Geometry: final body of the model. Coordinates: model frame, mm. A direction names the side the tool comes from. Give positions to 0.01 mm unless a question says otherwise; leave off trailing zeros. Write each loop counter-clockwise with the first axis right and the second up, starting at its lowest first coordinate (ties: lowest second). Pieces come first, ordered by that corner, then holes. Notation, with made-up numbers: (77.25, 84.25) -> (102.25, 84.25) arc R23 cw to (102.25, 123.25) -> close; hole circle Ø9 at (84.25, -26.75). An arc over 180 degrees is marked (long way). Answer as a JSON object with one key per item and string values.
Autodesk Fusion 360 part; units mm, degrees
sketch "Skizze1" plane through (0, 0, 0) normal (0, 1, 0) x (1, 0, 0)
  line L0 (14.5, -1) -> (-13.5, -1)
  line L1 (-13.5, -1) -> (-13.5, 0)
  line L2 (-13.5, 0) -> (14.5, 0)
  line L3 (14.5, 0) -> (14.5, -1)
  line L4 (14.5, -1) -> (-13.5, 0) construction
  line L5 (-13.5, -1) -> (14.5, 0) construction
  line L6 (-13.5, 0) -> (-12.5, 0)
  line L7 (-12.5, 0) -> (-12.5, -7.5)
  line L8 (-12.5, -7.5) -> (-13.5, -7.5)
  line L9 (-13.5, -7.5) -> (-13.5, 0)
  line L10 (14.5, 0) -> (13.5, 0)
  line L11 (13.5, 0) -> (13.5, -7.5)
  line L12 (13.5, -7.5) -> (14.5, -7.5)
  line L13 (14.5, -7.5) -> (14.5, 0)
  line L14 (-12.5, -7.5) -> (-16.15, -7.5)
  line L15 (-16.15, -7.5) -> (-16.15, -6.5)
  line L16 (-16.15, -6.5) -> (-12.5, -6.5)
  line L17 (-12.5, -6.5) -> (-12.5, -7.5)
  line L18 (13.5, -7.5) -> (17.15, -7.5)
  line L19 (17.15, -7.5) -> (17.15, -6.5)
  line L20 (17.15, -6.5) -> (13.5, -6.5)
  line L21 (13.5, -6.5) -> (13.5, -7.5)
  point P0 (0.5, -0.5)
  dimension "d7" = 28
  dimension "d8" = 1
  dimension "d9" = 7.5
  dimension "d10" = 1
  dimension "d11" = 7.5
  dimension "d12" = 1
  dimension "d13" = 3.65
  dimension "d14" = 1
  dimension "d15" = 3.65
  dimension "d16" = 1
extrude "Extrusion1" add sketch "Skizze1" along normal blind 200
fillet "Abrundung1" radius 1.5 4 edges at (13.5, 100, 7.5) (-12.5, 100, 7.5) (14.5, 100, 0) (-13.5, 100, 0)
fillet "Abrundung2" radius 0.5 4 edges at (-13.5, 100, 6.5) (14.5, 100, 6.5) (13.5, 100, 1) (-12.5, 100, 1)
sketch "Skizze2" plane through (0, 0, 1) normal (0, 0, 1) x (-1, 0, 0)
  line L0 (12, -200) -> (12, 0)
  line L1 (12, 0) -> (-13, 0)
  line L2 (-13, 0) -> (-13, -200)
  line L3 (-13, -200) -> (12, -200)
  line L4 (0, 0) -> (0, -4.15) construction
  line L5 (-2.05, -6.2) -> (-2.05, -13.8)
  arc A0 (-2.05, -13.8) -> (2.05, -13.8) centre (0, -13.8) ccw
  line L6 (2.05, -13.8) -> (2.05, -6.2)
  arc A1 (2.05, -6.2) -> (-2.05, -6.2) centre (0, -6.2) ccw
  line L7 (0, -4.15) -> (0, -15.85) construction
  point P0 (0, -4.15)
  dimension "d26" = 4.15
  dimension "d34" = 11.7
  dimension "d35" = 4.1
extrude "Extrusion2" cut sketch "Skizze2" against normal blind 1 contours L5 A0 L6 A1
pattern_linear "R-Anordnung1" count 10 spacing 20 along (0, 1, 0) of "Extrusion2"
equation "InnerWidth = 28 mm"
equation "OuterWidth = 35.3 mm"
equation "Height = 7.5 mm"
equation "Thickness = 1 mm"
equation "Length = 200 mm"
equation "SlotDistance = 25 mm"
equation "d7 = InnerWidth"
equation "d8 = Thickness"
equation "d9 = Height"
equation "d10 = Thickness"
equation "d11 = Height"
equation "d12 = Thickness"
equation "d13 = ( OuterWidth - InnerWidth ) / 2"
equation "d14 = Thickness"
equation "d15 = ( OuterWidth - InnerWidth ) / 2"
equation "d16 = Thickness"
equation "d17 = Length"
equation "OuterFillet = 1.5 mm"
equation "d20 = OuterFillet"
equation "InnerFillet = OuterFillet - Thickness"
equation "d22 = InnerFillet"
equation "SlotWidth = 4.1 mm"
equation "SlotLength = 11.7 mm"
equation "SlotDistance2 = 20 mm"
equation "d26 = Linear Dimension-2"
equation "d30 = Length / SlotDistance2"
equation "d32 = SlotDistance2"
equation "d34 = SlotLength"
equation "d35 = SlotWidth"
Q1. Cut plane B-B (y = 42). Return the cut outline in (x, z).
Values:
{"outline": "(-16.15, 6.5) -> (-14, 6.5) arc R0.5 cw to (-13.5, 6) -> (-13.5, 1.5) arc R1.5 ccw to (-12, 0) -> (13, 0) arc R1.5 ccw to (14.5, 1.5) -> (14.5, 6) arc R0.5 cw to (15, 6.5) -> (17.15, 6.5) -> (17.15, 7.5) -> (15, 7.5) arc R1.5 ccw to (13.5, 6) -> (13.5, 1.5) arc R0.5 cw to (13, 1) -> (-12, 1) arc R0.5 cw to (-12.5, 1.5) -> (-12.5, 6) arc R1.5 ccw to (-14, 7.5) -> (-16.15, 7.5) -> close"}
Q2. Cut plane A-A (z = 4.75). Return the cut outline in (x, y), and give its area (3 significant figures).
Values:
{"outline": "(-13.5, 0) -> (-12.5, 0) -> (-12.5, 200) -> (-13.5, 200) -> close; (13.5, 0) -> (14.5, 0) -> (14.5, 200) -> (13.5, 200) -> close", "area": "400 mm²"}
Q3. Material intervals for L1, parallel to X at y = 106, z = 3; L2, parallel to Z at x = 12, y = 126.5; L3, parallel to Z at x = -14, y = 78, sorted ascending. Write a range as from..to.
Values:
{"L1": "-13.5..-12.5, 13.5..14.5", "L2": "0..1", "L3": "6.5..7.5"}
Q4. Cut plane C-C (x = -9). Return the cut outline in (y, z), and give its area (3 significant figures).
Values:
{"outline": "(0, 0) -> (200, 0) -> (200, 1) -> (0, 1) -> close", "area": "200 mm²"}
Q5. Set-up query: faces 1 (the flat face through (0.4, 0, 0.7)), 2 (the flat face through (14.5, 99, 4)), 3 (the flat face through (1, 99, 1)). Return all of +Z, -Z, +X, -X, +Y, -Y with unobstructed straight access to the full face (end or side cutting, diameter ignored); none if empty.
Values:
{"face 1": "+Z, -Z, +X, -X, -Y", "face 2": "-Z, +X, +Y, -Y", "face 3": "+Z, +Y, -Y"}
Q6. Cut plane D-D (x = 0). State how many separate pieces and enclosed holes the cut face has, and give its area (3 significant figures).
Values:
{"separate pieces": "11", "enclosed holes": "0", "area": "83.0 mm²"}
Q7. First-contact query: P1, Ø0.8, axis at y = 51.5, z = 0.5, coming from the -X side; P2, Ø1.7, axis at x = -15.5, y = 62.5, coming from the -Z side; P3, Ø0.5, axis at y = 91, z = 0.5, coming from the -X side; P4, Ø12, axis at x = 3.5, y = 58, coming from the -Z side. Flat tips, straight axial feed; report the tip coordinate or a pass-through.
Values:
{"P1": "x = -13.37", "P2": "z = 6.5", "P3": "x = -13.3", "P4": "z = 0"}
Q8. Mould query, pull axis X, two halves, no side actions, for faces 4 (the flat face through (0.4, 200, 0.7)), 5 (the flat face through (13.5, 99, 4)), 6 (the flat face through (-13.5, 99, 4)). Classes: pulls with the +X half, pulls with the -X half, needs draft (parallel to the pull), parting line crosses it, or undercut.
Values:
{"face 4": "needs draft", "face 5": "undercut", "face 6": "pulls with the -X half"}
